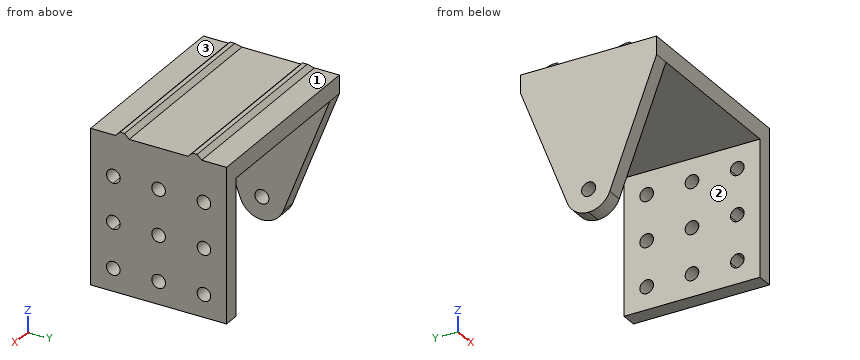
from build123d import *

# Parameters (mm, degrees)
F0_W          = 42
F0_H          = 30
F1_DEPTH      = 4
F2_W          = 3.5
F2_H          = 30
F3_DEPTH      = 30
F4_R          = 1.55
F5_DEPTH      = 5
F7_DEPTH      = 3.5
F8_W          = 42
F8_H          = 4
F9_DEPTH      = 1
F10_SIZE      = 1
F11_T4_DEPTH  = 48.7150489639
F11_T9_DEPTH  = 48.7150489639
F11_T14_DEPTH = 48.7150489639
F11_T19_DEPTH = 48.7150489639
F12_R         = 1.5
F13_DEPTH     = 3.5


# Not quite as in the source:
# - a fillet or chamfer that OpenCascade refuses, or shapes differently, is made with other operations: its cross-section is extruded or revolved along the edge and cut away or added


with BuildPart() as f1:
    # F0 (on Top) → F1 (new body)
    with BuildSketch(Plane.XY):
        Rectangle(F0_W, F0_H)
    extrude(amount=F1_DEPTH)

    # F2 (on face) → F3 (join)
    with BuildSketch(Plane(origin=(0, 0, 0), x_dir=(1, 0, 0), z_dir=(0, 0, -1))):
        with Locations((-19.25, 0)):
            Rectangle(F2_W, F2_H)
        with Locations((19.25, 0)):
            Rectangle(F2_W, F2_H)
    extrude(amount=F3_DEPTH)

    # F4 (on face) → F5 (cut)
    with BuildSketch(Plane(origin=(-21, 0, 0), x_dir=(0, -1, 0), z_dir=(-1, 0, 0))):
        with Locations((0, -25)):
            Circle(F4_R)
    extrude(amount=-F5_DEPTH, mode=Mode.SUBTRACT)

    # F6 (on face) → F7 (cut)
    with BuildSketch(Plane(origin=(-21, 0, 0), x_dir=(0, -1, 0), z_dir=(-1, 0, 0))):
        with BuildLine():
            ThreePointArc((0, -30), (-2.8288373248, -29.1228242007), (-4.665119593, -26.7990717558))
            Line((-4.665119593, -26.7990717558), (-15, 0))
            Line((-15, 0), (-15, -30))
            Line((-15, -30), (0, -30))
        make_face()
        with BuildLine():
            ThreePointArc((4.665119593, -26.7990717558), (2.8288373248, -29.1228242007), (0, -30))
            Line((0, -30), (15, -30))
            Line((15, -30), (15, 0))
            Line((15, 0), (4.665119593, -26.7990717558))
        make_face()
    extrude(amount=-F7_DEPTH, mode=Mode.SUBTRACT)

    # F8 (on face) → F9 (join)
    with BuildSketch(Plane.XY.offset(4)):
        with Locations((0, 8)):
            Rectangle(F8_W, F8_H)
        with Locations((0, -8)):
            Rectangle(F8_W, F8_H)
    extrude(amount=F9_DEPTH)

    # F10
    f10_edges = [f1.edges().sort_by_distance(p)[0] for p in [
        (-21, -8, 5),
        (-21, 8, 5),
    ]]
    chamfer(f10_edges, length=F10_SIZE)

    # F11: chamfer of 1.5 on 4 edges, made by hand


with BuildPart() as f11_tool2:
    # F11_s3 → F11_t4 (new body)
    with BuildSketch(Plane.YZ.offset(-23.8575244819)):
        Polygon((-8.5, 5), (-10, 3.5), (-10, 5), align=None)
    extrude(amount=F11_T4_DEPTH)

    split(bisect_by=Plane.XY.offset(4), keep=Keep.TOP)


with BuildPart() as f1_1:
    add(f1.part)

    # F11_t1: cut F11_tool2
    add(f11_tool2.part, mode=Mode.SUBTRACT)


with BuildPart() as f11_tool7:
    # F11_s8 → F11_t9 (new body)
    with BuildSketch(Plane.YZ.offset(24.8575244819)):
        Polygon((-6, 3.5), (-7.5, 5), (-6, 5), align=None)
    extrude(amount=-F11_T9_DEPTH)

    split(bisect_by=Plane.XY.offset(4), keep=Keep.TOP)


with BuildPart() as f1_2:
    add(f1_1.part)

    # F11_t6: cut F11_tool7
    add(f11_tool7.part, mode=Mode.SUBTRACT)


with BuildPart() as f11_tool12:
    # F11_s13 → F11_t14 (new body)
    with BuildSketch(Plane.YZ.offset(-23.8575244819)):
        Polygon((6, 3.5), (7.5, 5), (6, 5), align=None)
    extrude(amount=F11_T14_DEPTH)

    split(bisect_by=Plane.XY.offset(4), keep=Keep.TOP)


with BuildPart() as f1_3:
    add(f1_2.part)

    # F11_t11: cut F11_tool12
    add(f11_tool12.part, mode=Mode.SUBTRACT)


with BuildPart() as f11_tool17:
    # F11_s18 → F11_t19 (new body)
    with BuildSketch(Plane.YZ.offset(24.8575244819)):
        Polygon((10, 3.5), (8.5, 5), (10, 5), align=None)
    extrude(amount=-F11_T19_DEPTH)

    split(bisect_by=Plane.XY.offset(4), keep=Keep.TOP)


with BuildPart() as f1_4:
    add(f1_3.part)

    # F11_t16: cut F11_tool17
    add(f11_tool17.part, mode=Mode.SUBTRACT)

    # F12 (on face) → F13 (cut)
    with BuildSketch(Plane.YZ.offset(21)):
        with BuildLine():
            ThreePointArc((-10, -6.5), (-8.9393398282, -6.0606601718), (-8.5, -5))
            ThreePointArc((-8.5, -5), (-11.0606601718, -3.9393398282), (-10, -6.5))
        make_face()
        with BuildLine():
            ThreePointArc((-8.5, -25), (-8.9393398282, -23.9393398282), (-10, -23.5))
            ThreePointArc((-10, -23.5), (-11.0606601718, -26.0606601718), (-8.5, -25))
        make_face()
        with BuildLine():
            ThreePointArc((-8.5, -15), (-8.9393398282, -13.9393398282), (-10, -13.5))
            Line((-10, -13.5), (-10, -16.5))
            ThreePointArc((-10, -16.5), (-8.9393398282, -16.0606601718), (-8.5, -15))
        make_face()
        with BuildLine():
            Line((-10, -16.5), (-10, -13.5))
            ThreePointArc((-10, -13.5), (-11.5, -15), (-10, -16.5))
        make_face()
        with Locations((0, -5)):
            Circle(F12_R)
        with Locations((10, -5)):
            Circle(F12_R)
        with Locations((0, -15)):
            Circle(F12_R)
        with Locations((0, -25)):
            Circle(F12_R)
        with Locations((10, -15)):
            Circle(F12_R)
        with Locations((10, -25)):
            Circle(F12_R)
    extrude(amount=-F13_DEPTH, mode=Mode.SUBTRACT)


solid = f1_4.part
Geometry: final body of the model. Coordinates: model frame, mm. Face numbers are marked on the shaded views. A direction names the side the tool comes from. Give positions to 0.01 mm unless a question says otherwise; leave off trailing zeros. Order: outer loops, then holes, each group sorted by start corner. A loop starts at its lowest first (then second) coordinate and runs counter-clockwise, first axis right, second up. Notation, with made-up numbers: (-29, 57.25) - (7, 57.25) arc R11 cw to (7, 69.25) - close; hole circle Ø8 at (7.5, -27). An arc over 180 degrees is marked (long way). Use CSV: the item, a comma, the result in double quotes.
1. Section query A-A (x = 18). Give the number of separate pieces and of enclosed holes in the cut face, plus the area to 3 significant figures.
Answers below:
separate pieces,"1"
enclosed holes,"9"
area,"960 mm2"
2. Section query B-B (x = -10.5). Output: boundary loops of the cut face in (y, z), plus the area to 3 significant figures.
Answers below:
outline,"(-15, 0) - (15, 0) - (15, 4) - (9.5, 4) - (8.5, 5) - (7.5, 5) - (6.5, 4) - (-6.5, 4) - (-7.5, 5) - (-8.5, 5) - (-9.5, 4) - (-15, 4) - close"
area,"124 mm2"
3. Section query C-C (y = -4). Output: boundary loops of the cut face in (x, z).
Answers below:
outline,"(-21, -28) - (-17.5, -28) - (-17.5, 0) - (17.5, 0) - (17.5, -30) - (21, -30) - (21, 4) - (-21, 4) - close"
4. Material intervals for line 1 along Z through (x, y) = (19.15, 0); line 2 along X through (y, z) = (2.5, -14.5); line 3 along Z through (x, y) = (-9, -13.5), sorted ascending. Write a range as from..to.
Answers below:
line 1,"-30..-26.5, -23.5..-16.5, -13.5..-6.5, -3.5..4"
line 2,"-21..-17.5, 17.5..21"
line 3,"0..4"
5. Access query for the marked faces 1, 2 and 3. Directions: +Z, -Z, +X, -X, +Y, -Y. A direction counts if a zero-diameter tool reaches every point of the face in a straight line with its end or side. Return the directions, or none.
Answers below:
face 1,"+Z, +X, -X, +Y"
face 2,"-Z, +Y, -Y"
face 3,"+Z, +X, -X, -Y"
6. Contact query for flat-ended pins moving along their axis: pin 1 (2.5 mm diameter, centred on x = 0.5, y = -13.5, fed in from +Z); pin 2 (4 mm diameter, centred on y = 10, z = -15, fed in from +X); pin 3 (1.8 mm diameter, centred on y = 0, z = -15, fed in from +X); pin 4 (10 mm diameter, centred on x = 5.5, y = -0.5, fed in from -Z). Output: stop coordinate, or through.
Answers below:
pin 1,"z = 4"
pin 2,"x = 21"
pin 3,"x = -17.5"
pin 4,"z = 0"
7. Section query D-D (y = 10). Output: boundary loops of the cut face in (x, z), plus the area to 3 significant figures.
Answers below:
outline,"(-21, -12.97) - (-17.5, -12.97) - (-17.5, 0) - (17.5, 0) - (17.5, -3.5) - (21, -3.5) - (21, 4) - (-21, 4) - close; (17.5, -30) - (21, -30) - (21, -26.5) - (17.5, -26.5) - close; (17.5, -23.5) - (21, -23.5) - (21, -16.5) - (17.5, -16.5) - close; (17.5, -13.5) - (21, -13.5) - (21, -6.5) - (17.5, -6.5) - close"
area,"287 mm2"
